Work out the finished part from the listing and answer in its coordinate system (mm). Give positions to 0.01 mm unless a question says otherwise; leave off trailing zeros. Order: outer loops, then holes, each group sorted by start corner. A loop starts at its lowest first (then second) coordinate and runs counter-clockwise, first axis right, second up. Notation, with made-up numbers: (83.25, -11.5) -> (87.25, -11.5) arc R18 ccw to (87.25, -7.5) -> close; hole circle Ø4 at (-26, 29). An arc over 180 degrees is marked (long way). Use a Markdown table: item, result. Add a question column.
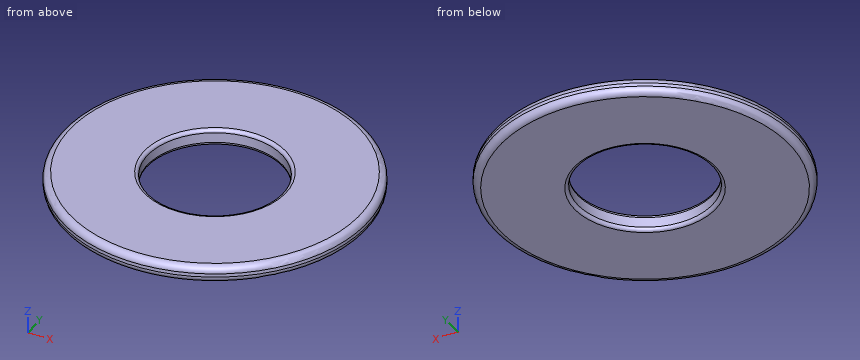
Autodesk Inventor part; units mm, degrees
ref_plane "YZ Plane" through (0, 0, 0) normal (1, 0, 0) x (0, 1, 0)
ref_plane "XZ Plane" through (0, 0, 0) normal (0, 1, 0) x (-1, 0, 0)
ref_plane "XY Plane" through (0, 0, 0) normal (0, 0, 1) x (1, 0, 0)
sketch "Sketch1" plane through (0, 0, 0) normal (0, 0, 1) x (1, 0, 0)
  circle A0 centre (0, 0) radius 2
  circle A1 centre (0, 0) radius 4.5
  dimension "Di" = 4
  dimension "D" = 9
extrude "Extrusion1" add sketch "Sketch1" along normal mid plane 0.5
fillet "Fillet1" radius 0.2 2 edges at (-4.5, 0, 0.25) (-4.5, 0, -0.25)
fillet "Fillet2" radius 0.1 2 edges at (-2, 0, 0.25) (-2, 0, -0.25)
properties part number "Anilha_M4"
1) The part is cut by section A-A, the plane y = 0. Determine the outline of the cut face in (x, z).
2) Straight lines are drawn through the part: line 1 (Y direction, x = 0, z = -0.05); line 2 (Y direction, x = -1.25, z = 0.1); line 3 (X direction, y = 2.75, z = 0.15). For each, find the intervals that lie inside material, in ascending order.
A:
| question | item | result |
|---|---|---|
| 1 | outline | (-4.5, -0.05) arc R0.2 ccw to (-4.3, -0.25) -> (-2.1, -0.25) arc R0.1 ccw to (-2, -0.15) -> (-2, 0.15) arc R0.1 ccw to (-2.1, 0.25) -> (-4.3, 0.25) arc R0.2 ccw to (-4.5, 0.05) -> close; (2, -0.15) arc R0.1 ccw to (2.1, -0.25) -> (4.3, -0.25) arc R0.2 ccw to (4.5, -0.05) -> (4.5, 0.05) arc R0.2 ccw to (4.3, 0.25) -> (2.1, 0.25) arc R0.1 ccw to (2, 0.15) -> close |
| 2 | line 1 | -4.5 to -2, 2 to 4.5 |
| 2 | line 2 | -4.32 to -1.56, 1.56 to 4.32 |
| 2 | line 3 | -3.53 to 3.53 |
